The model under review builds one solid part; all positions refer to its coordinate system, in mm. A direction names the side the tool comes from. Coordinates: 2 decimals unless noted, no trailing zeros. Loops run counter-clockwise (first coordinate to the right, second up) from the corner with the lowest first, then second, coordinate; pieces in that order, holes last. Notation, with made-up numbers: (31, 12) -> (61, 12) arc R17 ccw to (61, 40) -> close; hole circle Ø8 at (22.5, -28.75). An arc over 180 degrees is marked (long way). One line per question, with ' | ' between items. Start each with the question number.
from build123d import *

# Parameters (mm, degrees)
ESQUISSE1_R             = 57.5
ESQUISSE1_R_2           = 47.5
BOSS_EXTRU_1_DEPTH      = 10
ESQUISSE3_R             = 2.5
BOSS_EXTRU_2_DEPTH      = 10
ESQUISSE10_W            = 120
ESQUISSE10_H            = 120
BOSS_EXTRU_3_DEPTH      = 40
COQUE1_START            = 15
COQUE1_OUTLINE_W        = 110
COQUE1_OUTLINE_H        = 110
COQUE1_DEPTH            = 35
ESQUISSE14_R            = 47.5
ENL_V_MAT_EXTRU_1_DEPTH = 40


# Read off the part's stored shape, not the designer's step: Coque1
with BuildPart() as part:
    # Esquisse1 → Boss.-Extru.1 (new body)
    with BuildSketch(Plane(origin=(0, 0, 0), x_dir=(1, 0, 0), z_dir=(0, 1, 0))):
        with Locations(Location((0, 0, 0), (0, 0, 270))):
            Circle(ESQUISSE1_R)
        with Locations(Location((0, 0, 0), (0, 0, 270))):
            Circle(ESQUISSE1_R_2, mode=Mode.SUBTRACT)
    extrude(amount=BOSS_EXTRU_1_DEPTH)

    # Esquisse3 → Boss.-Extru.2 (add)
    with BuildSketch(Plane(origin=(0, 0, 0), x_dir=(1, 0, 0), z_dir=(0, 1, 0))):
        with Locations(Location((0, 52.5, 0), (0, 0, 270))):
            Circle(ESQUISSE3_R)
        with Locations(Location((0, -52.5, 0), (0, 0, 270))):
            Circle(ESQUISSE3_R)
        with Locations(Location((52.5, 0, 0), (0, 0, 270))):
            Circle(ESQUISSE3_R)
        with Locations(Location((-52.5, 0, 0), (0, 0, 270))):
            Circle(ESQUISSE3_R)
    extrude(amount=-BOSS_EXTRU_2_DEPTH)

    # Esquisse10 → Boss.-Extru.3 (add)
    with BuildSketch(Plane(origin=(0, 10, 0), x_dir=(1, 0, 0), z_dir=(0, 1, 0))):
        Rectangle(ESQUISSE10_W, ESQUISSE10_H)
    extrude(amount=BOSS_EXTRU_3_DEPTH)

    # Coque1 outline → Coque1 (cut)
    with BuildSketch(Plane(origin=(0, 0, 0), x_dir=(1, 0, 0), z_dir=(0, 1, 0)).offset(COQUE1_START)):
        Rectangle(COQUE1_OUTLINE_W, COQUE1_OUTLINE_H)
    extrude(amount=COQUE1_DEPTH, mode=Mode.SUBTRACT)

    # Esquisse14 → Enlèv. mat.-Extru.1 (cut)
    with BuildSketch(Plane.XZ.offset(-10)):
        with Locations(Location((0, 0, 0), (0, 0, 270))):
            Circle(ESQUISSE14_R)
    extrude(amount=-ENL_V_MAT_EXTRU_1_DEPTH, mode=Mode.SUBTRACT)


solid = part.part
1) Insertion check: pin 1 Ø1 at (x, y) = (37.5, 5) entering from -Z; pin 2 Ø5 at (y, z) = (5, 3.5) entering from -X. Each pin has a flat end and moves straight along its axis. Give the tip position at first contact, or say it passes through.
2) Mouldability with a two-part tool opening along X and no side actions: class faces 1 (the face through (-56.133, 4.93, -12.465)), 2 (the face through (-1, 32, -55)), 3 (the face through (-5, 50, 57)), 4 (the face through (50.06, -4.93, -0.54)) as +X half, -X half, draft (parallel to the pull), parting line (faces both ways), or undercut.
3) Consider section A-A, the plane y = 28.5. Write out the cut boundary in (x, z).
4) Machinability: for faces 5 (the face through (-52, -10, 0)), 6 (the face through (-1, 32, 55)), 7 (the face through (-0.96, -4.93, -50.19)), which of the approach directions +Z, -Z, +X, -X, +Y, -Y give a long, thin tool a straight path to every point of the face, cutting with its end or side? Answer none if there is none.
5) Consider section C-C, the plane x = 34. Write out the cut boundary in (y, z), plus the area to 3 significant figures.
6) Consider section B-B, the plane z = 0. Write out the cut boundary in (x, y), plus the area to 3 significant figures.
7) Wall thickness on L1, parallel to X at y = 37, z = -50.5; L2, parallel to X at y = 12.45, z = 0: over which ranges is each line inside the solid? List them lowest first.
8) Consider section D-D, the plane x = -44.5. Write out the cut boundary in (y, z).
Filled sheet:
1) pin 1: z = -44.01 | pin 2: x = -57.49
2) face 1: parting line | face 2: undercut | face 3: draft | face 4: undercut
3) outline: (-60, -60) -> (60, -60) -> (60, 60) -> (-60, 60) -> close; hole (-55, -55) -> (55, -55) -> (55, 55) -> (-55, 55) -> close
4) face 5: +Z, -Z, +X, -X, -Y | face 6: +Y | face 7: -Y
5) outline: (0, -46.37) -> (10, -46.37) -> (10, -60) -> (50, -60) -> (50, -55) -> (15, -55) -> (15, -33.17) -> (0, -33.17) -> close; (0, 33.17) -> (15, 33.17) -> (15, 55) -> (50, 55) -> (50, 60) -> (10, 60) -> (10, 46.37) -> (0, 46.37) -> close | area: 882 mm^2
6) outline: (-60, 10) -> (-57.5, 10) -> (-57.5, 0) -> (-55, 0) -> (-55, -10) -> (-50, -10) -> (-50, 0) -> (-47.5, 0) -> (-47.5, 15) -> (-55, 15) -> (-55, 50) -> (-60, 50) -> close; (47.5, 0) -> (50, 0) -> (50, -10) -> (55, -10) -> (55, 0) -> (57.5, 0) -> (57.5, 10) -> (60, 10) -> (60, 50) -> (55, 50) -> (55, 15) -> (47.5, 15) -> close | area: 775 mm^2
7) L1: -60 to -55, 55 to 60 | L2: -60 to -47.5, 47.5 to 60
8) outline: (0, -36.41) -> (10, -36.41) -> (10, -60) -> (50, -60) -> (50, -55) -> (15, -55) -> (15, -16.61) -> (0, -16.61) -> close; (0, 16.61) -> (15, 16.61) -> (15, 55) -> (50, 55) -> (50, 60) -> (10, 60) -> (10, 36.41) -> (0, 36.41) -> close
